from build123d import *

# Parameters (mm, degrees)
RESSALTO_EXTRUS_O1_DEPTH = 130
CHANFRO1_SIZE            = 30
CORTE_EXTRUS_O1_DEPTH    = 50
ESBO_O5_R                = 15
CORTE_EXTRUS_O2_DEPTH    = 293.06163733
CASCA1_T                 = 10


with BuildPart() as part:
    # Esboço1 → Ressalto-extrusão1 (new body)
    with BuildSketch(Plane(origin=(0, 0, 0), x_dir=(1, 0, 0), z_dir=(0, 1, 0))):
        Polygon((0, 120), (-103.923048454, 60), (-103.923048454, -60), (0, -120), (103.923048454, -60), (103.923048454, 60), align=None)
    extrude(amount=-RESSALTO_EXTRUS_O1_DEPTH)

    # Chanfro1
    chanfro1_edges = [part.edges().sort_by_distance(p)[0] for p in [
        (-103.923048454, -130, 0),
        (-51.961524227, -130, 90),
        (51.961524227, -130, 90),
        (103.923048454, -130, 0),
        (51.961524227, -130, -90),
        (-51.961524227, -130, -90),
    ]]
    chamfer(chanfro1_edges, length=CHANFRO1_SIZE)

    # Esboço2 → Corte-extrusão1 (cut)
    with BuildSketch(Plane(origin=(0, 0, 0), x_dir=(1, 0, 0), z_dir=(0, 1, 0))):
        Polygon((0, 108.452994616), (-93.923048454, 54.226497308), (-93.923048454, -54.226497308), (0, -108.452994616), (93.923048454, -54.226497308), (93.923048454, 54.226497308), align=None)
    extrude(amount=-CORTE_EXTRUS_O1_DEPTH, mode=Mode.SUBTRACT)

    # Esboço5 → Corte-extrusão2 (cut, through all)
    with BuildSketch(Plane(origin=(-51.961524227, 0, 90), x_dir=(0.8660254037844417, 0, 0.49999999999999495), z_dir=(-0.49999999999999495, 0, 0.8660254037844417))):
        with Locations((0, -30)):
            Circle(ESBO_O5_R)
    extrude(amount=-CORTE_EXTRUS_O2_DEPTH, mode=Mode.SUBTRACT)

    # Corte de superfície1
    split(bisect_by=Plane(origin=(0, -50, 0), x_dir=(1, 0, 0), z_dir=(0, 1, 0)), keep=Keep.BOTTOM)

    # Corte de superfície2
    split(bisect_by=Plane(origin=(0, -100, 0), x_dir=(1, 0, 0), z_dir=(0, 1, 0)), keep=Keep.BOTTOM)

    # Casca1 (no face opened: a closed hollow body)
    add(offset(amount=-CASCA1_T, mode=Mode.PRIVATE), mode=Mode.SUBTRACT)


solid = part.part
Read the model definition and answer for the solid it produces. Units are mm, in the model's axes. A direction names the side the tool comes from. Coordinates: 2 decimals unless noted, no trailing zeros. Loops run counter-clockwise (first coordinate to the right, second up) from the corner with the lowest first, then second, coordinate; pieces in that order, holes last. Notation, with made-up numbers: (54.25, 40.5) -> (105.25, 40.5) arc R19 ccw to (105.25, 58.5) -> close; hole circle Ø2 at (-25, 87). An arc over 180 degrees is marked (long way). Write item = value, one per line. Start each with the question number.
1) The part is cut by section B-B, the plane z = 76.5. Determine the outline of the cut face in (x, y).
2) Given P1, Ø6, axis at y = -109.5, z = -18.5, coming from the -X side; P2, Ø2, axis at y = -114, z = 28, coming from the +X side; P3, Ø1, axis at y = -124.5, z = -20.5, coming from the -X side, each flat-ended and moving along its own axis, determine where each tip first touches the part or whether it passes through.
3) Find the intervals of material crossed by L1, parallel to Y at x = -38, z = -31.5; L2, parallel to Z at x = -58, y = -113; L3, parallel to X at y = -117, z = 67, in increasing order. Write a range as from..to.
4) The mould has two halves that part along X. Classify faces 1 (the face through (88.713, -115.21, 0.84)), 2 (the face through (-88.713, -115.21, -0.84)), 3 (the face through (-74.71, -115.07, -0.64)): pulls with the +X half, pulls with the -X half, needs draft (parallel to the pull), parting line crosses it, or undercut.
5) The part is cut by section C-C, the plane y = -106.5. Determine the outline of the cut face in (x, z).
6) The part is cut by section A-A, the plane x = 39. Determine the outline of the cut face in (y, z), plus the area to 3 significant figures.
7) For faces 4 (the face through (-43.63, -115.21, -77.25)), 5 (the face through (36.8, -115.07, 65.02)), determine the directions among +Z, -Z, +X, -X, +Y, -Y from which every point of the face is accessible in a straight line to the end or side of a thin tool.
8) The part is cut by section D-D, the plane z = -104. Determine the outline of the cut face in (x, y), plus the area to 3 significant figures.
Result:
q1.outline = (-75.34, -100) -> (-15.34, -130) -> (15.34, -130) -> (75.34, -100) -> close; hole (-27.06, -110) -> (-7.06, -120) -> (7.06, -120) -> (27.06, -110) -> close
q2.P1 = -97.42
q2.P2 = 90.92
q2.P3 = -79.92
q3.L1 = -130..-120, -110..-100
q3.L2 = -71.5..-55.17, 55.17..71.5
q3.L3 = -57.8..-29.51, 29.51..57.8
q4.face_1 = pulls with the +X half
q4.face_2 = pulls with the -X half
q4.face_3 = undercut
q5.outline = (-97.42, -56.25) -> (0, -112.49) -> (97.42, -56.25) -> (97.42, 56.25) -> (0, 112.49) -> (-97.42, 56.25) -> close
q6.outline = (-130, -62.84) -> (-100, -97.48) -> (-100, 97.48) -> (-130, 62.84) -> close; hole (-120, -58.06) -> (-110, -69.61) -> (-110, 69.61) -> (-120, 58.06) -> close
q6.area = 3,530 mm²
q7.face_4 = -Z, -X, -Y
q7.face_5 = none
q8.outline = (-27.71, -100) -> (0, -113.86) -> (27.71, -100) -> close
q8.area = 384 mm²
